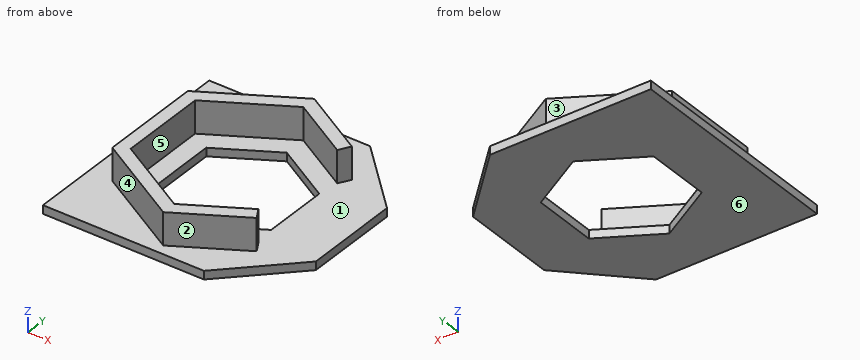
```python
from build123d import *

# Parameters (mm, degrees)
F0_W     = 35
F0_H     = 35
F1_DEPTH = 1.3
F3_DEPTH = 25
F4_DEPTH = 5
F5_SIZE  = 10


with BuildPart() as f1:
    # F0 (on Top) → F1 (new body)
    with BuildSketch(Plane.XY):
        with Locations((17.5, 17.5)):
            Rectangle(F0_W, F0_H)
    extrude(amount=F1_DEPTH)

    # F2 (on face) → F3 (cut)
    with BuildSketch(Plane.XY.offset(1.3)):
        Polygon((26.275, 22.566249), (17.5, 27.632497), (8.725, 22.566249), (8.725, 12.433751), (17.5, 7.367503), (26.275, 12.433751), align=None)
    extrude(amount=-F3_DEPTH, mode=Mode.SUBTRACT)

    # F2 (on face) → F4 (join)
    with BuildSketch(Plane.XY.offset(1.3)):
        Polygon((5.725, 10.701701), (5.725, 24.298299), (17.5, 31.096599), (26.676924, 25.798299), (27.676924, 27.53035), (17.5, 33.406), (3.725, 25.453), (3.725, 9.547), (17.5, 1.594), (27.676924, 7.46965), (26.676924, 9.201701), (17.5, 3.903401), align=None)
    extrude(amount=F4_DEPTH)

    # F5
    f5_edges = [f1.edges().sort_by_distance(p)[0] for p in [
        (35, 0, 0.65),
        (35, 35, 0.65),
    ]]
    chamfer(f5_edges, length=F5_SIZE)


solid = f1.part
```
Geometry: final body of the model. Coordinates: model frame, mm. Face numbers are marked on the shaded views. A direction names the side the tool comes from. Coordinates: 2 decimals unless noted, no trailing zeros. Order: outer loops, then holes, each group sorted by start corner. A loop starts at its lowest first (then second) coordinate and runs counter-clockwise, first axis right, second up.
Item 1: Section query C-C (y = 28.5). Output: boundary loops of the cut face in (x, z), then the cut area to 4 significant figures.
Answer:
outline: (0, 0) - (31.5, 0) - (31.5, 1.3) - (26, 1.3) - (26, 6.3) - (22, 6.3) - (22, 1.3) - (13, 1.3) - (13, 6.3) - (9, 6.3) - (9, 1.3) - (0, 1.3) - close
area: 80.95 mm2
Item 2: Section query B-B (z = 5). Output: boundary loops of the cut face in (x, y) (3 decimals), then the cut area to 3 significant figures.
Answer:
outline: (3.725, 9.547) - (17.5, 1.594) - (27.677, 7.47) - (26.677, 9.202) - (17.5, 3.903) - (5.725, 10.702) - (5.725, 24.298) - (17.5, 31.097) - (26.677, 25.798) - (27.677, 27.53) - (17.5, 33.406) - (3.725, 25.453) - close
area: 133 mm2
Item 3: Section query D-D (x = 4.5). Output: boundary loops of the cut face in (y, z).
Answer:
outline: (0, 0) - (35, 0) - (35, 1.3) - (25.9, 1.3) - (25.9, 6.3) - (9.1, 6.3) - (9.1, 1.3) - (0, 1.3) - close
Item 4: Section query A-A (x = 14). Output: boundary loops of the cut face in (y, z), then the cut area to 3 significant figures.
Answer:
outline: (0, 0) - (9.39, 0) - (9.39, 1.3) - (5.92, 1.3) - (5.92, 6.3) - (3.61, 6.3) - (3.61, 1.3) - (0, 1.3) - close; (25.61, 0) - (35, 0) - (35, 1.3) - (31.39, 1.3) - (31.39, 6.3) - (29.08, 6.3) - (29.08, 1.3) - (25.61, 1.3) - close
area: 47.5 mm2
Item 5: Contact query for flat-ended pins moving along their axis: P1, Ø2, axis at x = 23, z = 3, coming from the -Y side; P2, Ø1.5, axis at y = 20.5, z = 4, coming from the +X side (3 decimals); P3, Ø1.5, axis at y = 19.5, z = 4, coming from the -X side (3 decimals). Output: stop coordinate, or through.
Answer:
P1: stops at y = 4.19
P2: stops at x = 5.725
P3: stops at x = 3.725
Item 6: Material intervals for line 1 along Z through (x, y) = (12, 25.5); line 2 along X through (y, z) = (26, 2.5); line 3 along Y through (x, z) = (14, 3), sorted ascending.
Answer:
line 1: z = 0 to 1.3
line 2: x = 4.67 to 8.67, 26.33 to 26.79
line 3: y = 3.61 to 5.92, 29.08 to 31.39
Item 7: Draft query along Y for the marked faces 4, 5 and 6. Return one class per face: released by +Y, released by -Y, zero draft, split by the parting line, or undercut.
Answer:
face 4: released by -Y
face 5: undercut
face 6: zero draft
Item 8: Access query for the marked faces 1, 2 and 3. Directions: +Z, -Z, +X, -X, +Y, -Y. A direction counts if a zero-diameter tool reaches every point of the face in a straight line with its end or side. Return the directions, or none.
Answer:
face 1: +Z
face 2: +Z, +X, -Y
face 3: +Z, -X, +Y
